Autodesk Fusion 360 part; units mm, degrees
sketch "スケッチ1" plane through (0, 0, 0) normal (0, 0, 1) x (1, 0, 0)
  line L0 (0, 10) -> (-5, 10)
  line L1 (-5, 10) -> (-5, -15)
  line L2 (-5, -15) -> (0, -15)
  line L3 (0, -15) -> (0, 10)
  dimension "d1" = 25
  dimension "d2" = 5
  dimension "d3" = 10
extrude "押し出し1" add sketch "スケッチ1" against normal blind 24
sketch "スケッチ2" plane through (0, 0, 0) normal (1, 0, 0) x (0, 1, 0)
  line L0 (10, 0) -> (-15, 0)
  line L1 (-15, 0) -> (-15, -24)
  line L2 (-15, -24) -> (10, -24)
  line L3 (10, -24) -> (10, 0)
  line L4 (0, 0) -> (0, -24) construction
  circle A0 centre (0, -7.5) radius 2.7
  circle A1 centre (0, -7.5) radius 4.7
  line L5 (-9, 0) -> (-9, -24)
  line L6 (-15, -14) -> (-9, -14)
  line L7 (-4, -24) -> (-4, -12.5)
  line L8 (-4, -12.5) -> (4, -12.5)
  line L9 (4, -12.5) -> (4, -24)
  dimension "d6" = 5.4
  dimension "d7" = 9.4
  dimension "d8" = 7.5
  dimension "d9" = 6
  dimension "d10" = 10
  dimension "d19" = 8
  dimension "d20" = 4
  dimension "d21" = 11.5
extrude "押し出し2" cut sketch "スケッチ2" against normal up to surface (5 mm away) contours A0
extrude "押し出し3" cut sketch "スケッチ2" against normal blind 3 contours A1
extrude "押し出し4" add sketch "スケッチ2" along normal blind 6.5 contours L1 L2 L5 L6
chamfer "面取り1" distance 14 distance2 6.5 1 edges at (0, -12, -14) measured on face at (0, 0.4504, -20.0623)
extrude "押し出し5" add sketch "スケッチ2" against normal blind 6.5 contours L2 L7 L8 L9
sketch "スケッチ3" plane through (0, 0, 0) normal (0, 0, 1) x (-1, 0, 0)
  line L0 (0, 15) -> (0, 9)
  line L1 (0, 9) -> (0, -10)
  line L2 (0, -10) -> (5, -10)
  line L3 (5, -10) -> (5, 15)
  line L4 (5, 15) -> (0, 15)
  line L5 (0, 0) -> (-3, 0) construction
  circle A0 centre (-3, 0) radius 7.6
  circle A1 centre (-3, 0) radius 6
  dimension "d24" = 3
  dimension "d25" = 15.2
  dimension "d26" = 12
extrude "押し出し6" cut sketch "スケッチ3" against normal blind 3.6 from surface at -12 contours L1 A0 A1 picked at (0.3272, 6.2175)
hole "穴1" at (3, -15, -19) direction (0, 1, 0) diameter 2.5 depth 6 tip angle 118
fillet "フィレット1" radius 0.5 7 edges at (-5, 10, -12) (0, 10, -12) (3.25, -9, -7) (6.5, -9, -19) (3.25, -15, -7) (6.5, -15, -19) (-5, -15, -12)
equation "d20 = d19 / 2"
Geometry check sheet. Reference: the model listing, model coordinates, mm. A direction names the side the tool comes from. Give positions to 0.01 mm unless a question says otherwise; leave off trailing zeros. Loops run counter-clockwise (first coordinate to the right, second up) from the corner with the lowest first, then second, coordinate; pieces in that order, holes last. Notation, with made-up numbers: M 39.25,-2.75 L 76.25,-2.75 A16 cw 76.25,14.25 Z; hole C 47,59.5 d5. An arc over 180 degrees is marked long. Answer as CSV lines item,"result".
Item 1: Material ranges on line 1 (Z direction, x = -4.4, y = 0); line 2 (Z direction, x = -1.65, y = 0); line 3 (X direction, y = -10.55, z = -19), recorded low to high.
Values:
line 1,"z = -24 to -15.6, -12 to -10.2, -4.8 to 0"
line 2,"z = -24 to -12.2, -2.8 to 0"
line 3,"x = -5 to 1.75, 4.25 to 6.5"
Item 2: Cross-section at C-C on x = -2.5. Record the cut outline in (y, z) (3 decimals), and give its area (3 significant figures).
Values:
outline,"M -15,-24 L 10,-24 L 10,0 L -15,0 Z; hole M -5.245,-15.6 L -2.398,-15.6 L -2.398,-12 L -5.245,-12 Z; hole C 0,-7.5 d9.4; hole M 2.398,-15.6 L 5.245,-15.6 L 5.245,-12 L 2.398,-12 Z"
area,"510 mm²"
Item 3: Depth check by flat-ended pin: P1, Ø0.8, axis at x = -5.5, y = 1, coming from the +Z side; P2, Ø1, axis at y = -0.5, z = -4, coming from the +X side; P3, Ø7.5, axis at y = -1, z = -5.5, coming from the +X side. Enter the tip coordinate at first touch or a pass-through.
Values:
P1,"stops at z = -12.5"
P2,"stops at x = -3"
P3,"stops at x = 0"
Item 4: Access from +Z, -Z, +X, -X, +Y, -Y to the whole of each face (thin tool, end or side, straight path). Record for faces 4 (the flat face through (-6, 0, -12.5)), 5 (the flat face through (-3.3, -0.1, -15.6)), 6 (the flat face through (-6, 4, -18)).
Values:
face 4,"+Z, -X, +Y, -Y"
face 5,"none"
face 6,"+Z, -Z, -X, +Y"
Item 5: Release check for a two-part mould opening along X. For faces 1 (the cylindrical face through (-3, 0, -14)), 2 (the flat face through (-3, -2, 0)), 3 (the flat face through (-3, -2.2, -9.4)) record: pulls with the +X half, pulls with the -X half, needs draft (parallel to the pull), parting line crosses it, or undercut.
Values:
face 1,"undercut"
face 2,"needs draft"
face 3,"pulls with the +X half"
Item 6: Cross-section at A-A on y = 0. Record the cut outline in (x, z), and give its area (3 significant figures).
Values:
outline,"M -6.5,-24 L 0,-24 L 0,-12.2 L -3,-12.2 L -3,-15.6 L -4.6,-15.6 L -4.6,-12 L -3,-12 L -3,-10.2 L -5,-10.2 L -5,-12.5 L -6.5,-12.5 Z; M -5,-4.8 L -3,-4.8 L -3,-2.8 L 0,-2.8 L 0,0 L -5,0 Z"
area,"92.5 mm²"
Item 7: Cross-section at D-D on y = -3.5. Record the cut outline in (x, z).
Values:
outline,"M -6.5,-24 L 0,-24 L 0,-10.64 L -3,-10.64 L -3,-4.36 L 0,-4.36 L 0,0 L -5,0 L -5,-12.5 L -6.5,-12.5 Z; hole M -3.75,-15.6 L -1.87,-15.6 L -1.87,-12 L -3.75,-12 Z"
Item 8: Cross-section at B-B on z = -19. Record the cut outline in (x, y).
Values:
outline,"M -6.5,-4 L -5,-4 L -5,-14.5 A0.5 ccw -4.5,-15 L 1.75,-15 L 1.75,-9 L 0,-9 L 0,9.5 A0.5 ccw -0.5,10 L -4.5,10 A0.5 ccw -5,9.5 L -5,4 L -6.5,4 Z; M 4.25,-15 L 6,-15 A0.5 ccw 6.5,-14.5 L 6.5,-9.5 A0.5 ccw 6,-9 L 4.25,-9 Z"
